from build123d import *

# Parameters (mm, degrees)
SKETCH_1_W      = 46
SKETCH_1_H      = 46
EXTRUDE_1_DEPTH = 3
SKETCH_3_R      = 5
EXTRUDE_2_DEPTH = 2
SKETCH_4_R      = 2.5
EXTRUDE_3_DEPTH = 1.5
FILLET_1_R      = 5
FILLET_2_R      = 2
SKETCH_5_W      = 3
SKETCH_5_H      = 15
SKETCH_5_W_2    = 15
SKETCH_5_H_2    = 3
EXTRUDE_4_DEPTH = 5
FILLET_3_R      = 2


with BuildPart() as part:
    # ｽｹｯﾁ1 → ﾎﾞｽ - 押し出し1 (new body)
    with BuildSketch(Plane.XY):
        with Locations((23, 23)):
            Rectangle(SKETCH_1_W, SKETCH_1_H)
    extrude(amount=EXTRUDE_1_DEPTH)

    # ｽｹｯﾁ3 → ﾎﾞｽ - 押し出し2 (add)
    with BuildSketch(Plane.XY.offset(3)):
        with Locations((23, 23)):
            Circle(SKETCH_3_R)
    extrude(amount=EXTRUDE_2_DEPTH)

    # ｽｹｯﾁ4 → ﾎﾞｽ - 押し出し3 (add)
    with BuildSketch(Plane.XY.offset(5)):
        with Locations((23, 23)):
            Circle(SKETCH_4_R)
    extrude(amount=EXTRUDE_3_DEPTH)

    # ﾌｨﾚｯﾄ1
    fillet_1_edges = [part.edges().sort_by_distance(p)[0] for p in [
        (0, 46, 1.5),
        (46, 46, 1.5),
        (46, 0, 1.5),
        (0, 0, 1.5),
    ]]
    fillet(fillet_1_edges, radius=FILLET_1_R)

    # ﾌｨﾚｯﾄ2
    fillet_2_edges = [part.edges().sort_by_distance(p)[0] for p in [
        (18, 23, 3),
    ]]
    fillet(fillet_2_edges, radius=FILLET_2_R - 0.0001)  # a hair under: the kernel refuses the full size

    # ｽｹｯﾁ5 → ﾎﾞｽ - 押し出し4 (add)
    with BuildSketch(Plane.XY.offset(3)):
        with Locations((4.5, 23)):
            Rectangle(SKETCH_5_W, SKETCH_5_H)
        with Locations((23, 41.5)):
            Rectangle(SKETCH_5_W_2, SKETCH_5_H_2)
        with Locations((41.5, 23)):
            Rectangle(SKETCH_5_W, SKETCH_5_H)
    extrude(amount=EXTRUDE_4_DEPTH)

    # ﾌｨﾚｯﾄ3
    fillet_3_edges = [part.edges().sort_by_distance(p)[0] for p in [
        (4.5, 30.5, 3),
        (3, 23, 3),
        (4.5, 15.5, 3),
        (15.5, 41.5, 3),
        (30.5, 41.5, 3),
        (23, 43, 3),
        (41.5, 15.5, 3),
        (43, 23, 3),
        (41.5, 30.5, 3),
    ]]
    fillet(fillet_3_edges, radius=FILLET_3_R)


solid = part.part
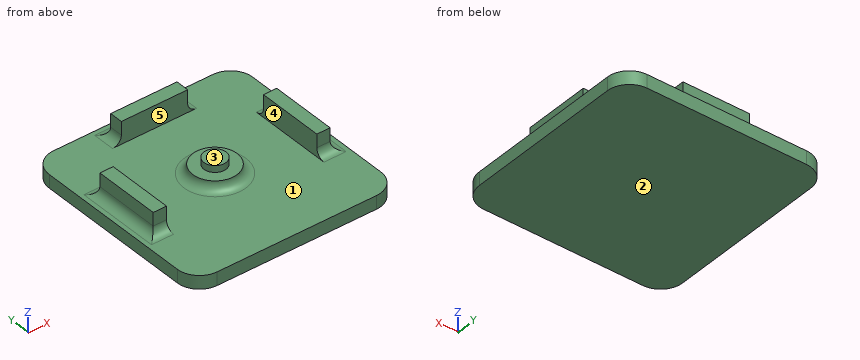
Design review of the part built by this model. Coordinates are the model's own, in mm. Face numbers are marked on the shaded views. A direction names the side the tool comes from. Coordinates: 2 decimals unless noted, no trailing zeros. Loops run counter-clockwise (first coordinate to the right, second up) from the corner with the lowest first, then second, coordinate; pieces in that order, holes last.
Item 1: Wall thickness on L1, parallel to X at y = 29, z = 5.5; L2, parallel to X at y = 25, z = 3.25; L3, parallel to Z at x = 32, y = 38: over which ranges is each line inside the solid? List them lowest first.
Completed:
L1: x = 3 to 6, 40 to 43
L2: x = 1.97 to 6, 17.31 to 28.69, 40 to 44.03
L3: z = 0 to 3
Item 2: Clearance check with flat-ended pins moving along their axes: pin 1 (2.5 mm diameter, centred on x = 4, z = 6.5, fed in from +Y); pin 2 (2.5 mm diameter, centred on x = 26.5, z = 6.5, fed in from -Y); pin 3 (3 mm diameter, centred on x = 21, y = 22.5, fed in from +Z); pin 4 (4 mm diameter, centred on x = 23, y = 22.5, fed in from -Z). State where each tip first meets the part, or that it passes through.
Completed:
pin 1: stops at y = 30.5
pin 2: stops at y = 21.91
pin 3: stops at z = 6.5
pin 4: stops at z = 0
Item 3: Add section D-D (x = 4). Write out the cut boundary in (y, z).
Completed:
outline: (0.1, 0) - (45.9, 0) - (45.9, 3) - (32.5, 3) arc R2 cw to (30.5, 5) - (30.5, 8) - (15.5, 8) - (15.5, 5) arc R2 cw to (13.5, 3) - (0.1, 3) - close
Item 4: Draft analysis for pull direction X (two halves, no side actions). For the marked faces 4 and 5, state which applies: pulls with the +X half, pulls with the -X half, needs draft (parallel to the pull), parting line crosses it, or undercut.
Completed:
face 4: undercut
face 5: needs draft
Item 5: For the marked faces 1, 2 and 3, list the 3-axis set-ups (+Z, -Z, +X, -X, +Y, -Y) from which the entire face can be reached by the end or side of a thin tool; tool diameter is ignored.
Completed:
face 1: +Z
face 2: -Z, +X, -X, +Y, -Y
face 3: +Z, -Y
Item 6: Add section A-A (z = 7.25). Write out the cut boundary in (x, y), and give its area (3 significant figures).
Completed:
outline: (3, 15.5) - (6, 15.5) - (6, 30.5) - (3, 30.5) - close; (15.5, 40) - (30.5, 40) - (30.5, 43) - (15.5, 43) - close; (40, 15.5) - (43, 15.5) - (43, 30.5) - (40, 30.5) - close
area: 135 mm2
